The figure shows three views and two pictorial views of one solid part (mm, origin at its lowest corner). Answer the questions. A direction names the side the tool comes from. Give positions to 0.01 mm unless a question says otherwise; leave off trailing zeros. Order: outer loops, then holes, each group sorted by start corner. A loop starts at its lowest first (then second) coordinate and runs counter-clockwise, first axis right, second up. Notation, with made-up numbers: M 1.5,85.5 L 34.5,85.5 A21 ccw 34.5,108.5 Z; hole C 13,-30.5 d4. An arc over 180 degrees is marked long. One line per item, written item: value.
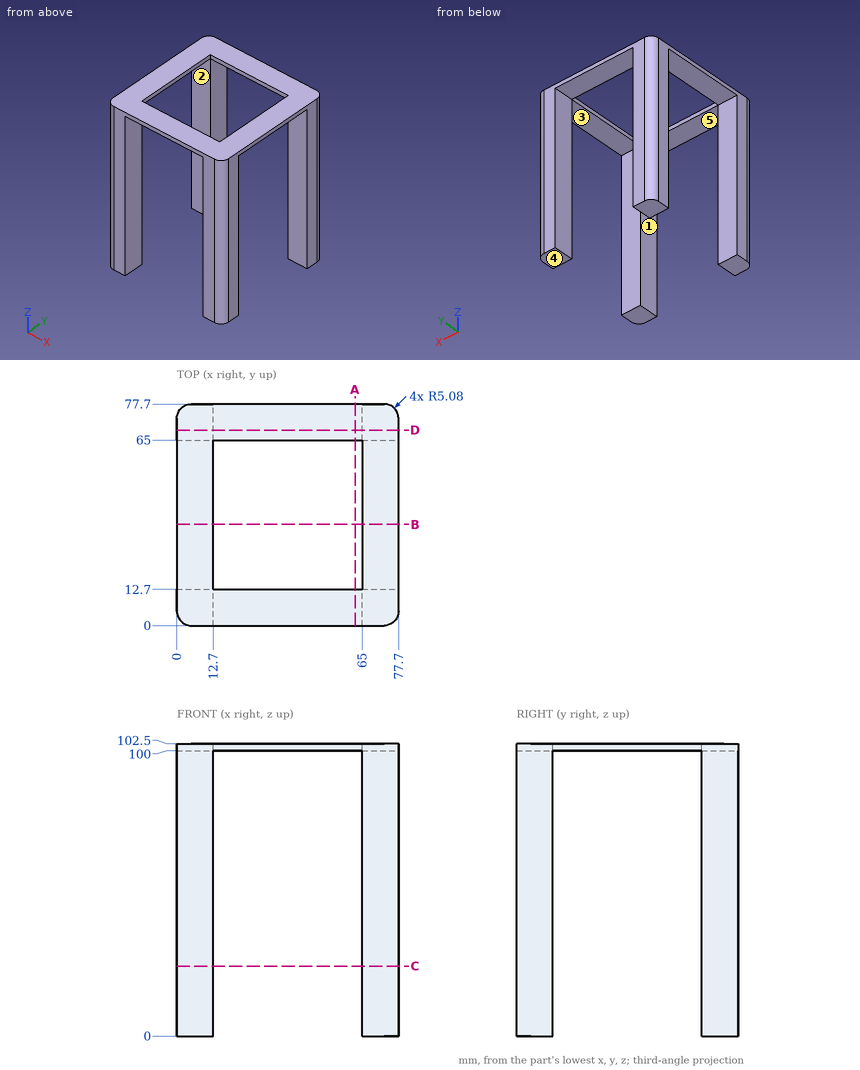
1) Find section C-C, the plane z = 24.5. Write down the section's boundary in (x, y), plus the area to 3 significant figures.
Reported:
outline: M 0,5.08 A5.08 ccw 5.08,0 L 12.7,0 L 12.7,12.7 L 0,12.7 Z; M 0,65 L 12.7,65 L 12.7,77.7 L 5.08,77.7 A5.08 ccw 0,72.62 Z; M 65,0 L 72.62,0 A5.08 ccw 77.7,5.08 L 77.7,12.7 L 65,12.7 Z; M 65,65 L 77.7,65 L 77.7,72.62 A5.08 ccw 72.62,77.7 L 65,77.7 Z
area: 623 mm^2
2) Find section D-D, the plane y = 68.5. Write down the section's boundary in (x, z).
Reported:
outline: M 0,0 L 12.7,0 L 12.7,100 L 65,100 L 65,0 L 77.7,0 L 77.7,102.5 L 0,102.5 Z
3) Consider probe 1 along Y at (x, z) = (73, 84); probe 2 along X at (y, z) = (68, 68); probe 3 along X at (y, z) = (74.5, 86). Determine where each line is inside the solid, lowest interval first.
Reported:
probe 1: y = 0.01 to 12.7, 65 to 77.69
probe 2: x = 0 to 12.7, 65 to 77.7
probe 3: x = 0.36 to 12.7, 65 to 77.34
4) Find section A-A, the plane x = 62.5. Write down the section's boundary in (y, z).
Reported:
outline: M 0,100 L 12.7,100 L 12.7,102.5 L 0,102.5 Z; M 65,100 L 77.7,100 L 77.7,102.5 L 65,102.5 Z
5) Determine the mould class of the marked faces 1 and 2 for opening direction Y: +Y half, -Y half, draft (parallel to the pull), parting line (faces both ways), or undercut.
Reported:
face 1: draft
face 2: undercut
6) Which of the six approach directions +Z, -Z, +X, -X, +Y, -Y give full straight-line access (tool end or side, diameter ignored) to the marked faces 3, 4 and 5?
Reported:
face 3: -Z, +X, -X
face 4: -Z, +X, -X, +Y, -Y
face 5: -Z, +Y, -Y
7) This flat-tipped pin is pushed along its axis until it touches: pin 1 Ø10 at (x, y) = (9.5, 44.5) entering from -Z. Where does it stop, or does it pass through?
Reported:
pin 1: stops at z = 100
